from build123d import *

# Parameters (mm, degrees)
SKETCH1_R           = 3
BOSS_EXTRUDE1_DEPTH = 1.5
SKETCH2_R           = 1.875
BOSS_EXTRUDE2_DEPTH = 15
CUT_EXTRUDE1_DEPTH  = 0.75
FILLET2_R           = 0.1


with BuildPart() as part:
    # Sketch1 → Boss-Extrude1 (new body)
    with BuildSketch(Plane.XY):
        Circle(SKETCH1_R)
    extrude(amount=BOSS_EXTRUDE1_DEPTH)

    # Sketch2 → Boss-Extrude2 (add)
    with BuildSketch(Plane.XY.offset(1.5)):
        Circle(SKETCH2_R)
    extrude(amount=BOSS_EXTRUDE2_DEPTH)

    # Sketch3 → Cut-Extrude1 (cut)
    with BuildSketch(Plane(origin=(0, 0, 0), x_dir=(-1, 0, 0), z_dir=(0, 0, -1))):
        with BuildLine():
            Line((2.977836652, 0.322793516), (-2.982583502, 0.322793516))
            ThreePointArc((-2.982583502, 0.322793516), (-3, 0), (-2.982583502, -0.322793516))
            ThreePointArc((-2.982583502, -0.322793516), (-2.980281261, -0.343400064), (-2.977836652, -0.363990208))
            Line((-2.977836652, -0.363990208), (2.977836652, -0.363990208))
            ThreePointArc((2.977836652, -0.363990208), (2.994454037, -0.182332173), (3, 0))
            ThreePointArc((3, 0), (2.995642711, 0.161631516), (2.982583502, 0.322793516))
            Line((2.982583502, 0.322793516), (2.977836652, 0.322793516))
        make_face()
    extrude(amount=-CUT_EXTRUDE1_DEPTH, mode=Mode.SUBTRACT)

    # Fillet2
    fillet2_edges = [part.edges().sort_by_distance(p)[0] for p in [
        (0, -0.363990208, 0.75),
        (0, 0.322793516, 0.75),
    ]]
    fillet(fillet2_edges, radius=FILLET2_R)


solid = part.part
Check sheet for the modelled part. Datum: model origin and axes. Units: mm. A direction names the side the tool comes from. Round coordinates to 2 decimals unless told otherwise and drop trailing zeros. Order: outer loops, then holes, each group sorted by start corner. A loop starts at its lowest first (then second) coordinate and runs counter-clockwise, first axis right, second up.
(1) Access from +Z, -Z, +X, -X, +Y, -Y to the whole of each face (thin tool, end or side, straight path). Record for faces 1 (the cylindrical face through (-1.873, 0.082, 8.895)), 2 (the flat face through (0, -1, 0)).
(2) Cross-section at A-A, the plane y = 0. Enter the section's corners in (x, z) (3 decimals), and give its area (4 significant figures).
(3) Scan lines: probe 1 along Z at (x, y) = (-1.5, 1.5); probe 2 along Z at (x, y) = (-1, 0.25); probe 3 along Y at (x, z) = (0.5, 14.75). Record each from-to range of solid material in increasing order.
(4) Cross-section at C-C, the plane z = 11.5. Enter the section's corners in (x, y) (3 decimals), and give its area (3 significant figures).
(5) Cross-section at D-D, the plane y = 1. Enter the section's corners in (x, z), and give its area (3 significant figures).
(6) Cross-section at B-B, the plane x = 0. Enter the section's corners in (y, z) (3 decimals).
(7) Go/stop test with flat-tipped pins: P1, Ø1, axis at x = -0.5, z = 6.5, coming from the +Y side (3 decimals); P2, Ø3, axis at y = 0.5, z = 11, coming from the +X side (3 decimals); P3, Ø1, axis at y = 1, z = 13, coming from the -X side. Record where each tip stops, or that it passes through.
Check sheet entries:
1. face 1: +Z
1. face 2: -Z, +X, -X, +Y, -Y
2. outline: (-3, 0.75) - (3, 0.75) - (3, 1.5) - (1.875, 1.5) - (1.875, 16.5) - (-1.875, 16.5) - (-1.875, 1.5) - (-3, 1.5) - close
2. area: 60.75 mm2
3. probe 1: z = 0 to 1.5
3. probe 2: z = 0.75 to 16.5
3. probe 3: y = -1.81 to 1.81
4. outline: circle Ø3.75 at (0, 0)
4. area: 11.0 mm2
5. outline: (-2.83, 0) - (2.83, 0) - (2.83, 1.5) - (1.59, 1.5) - (1.59, 16.5) - (-1.59, 16.5) - (-1.59, 1.5) - (-2.83, 1.5) - close
5. area: 56.1 mm2
6. outline: (-3, 0) - (-0.364, 0) - (-0.364, 0.65) arc R0.1 cw to (-0.264, 0.75) - (0.223, 0.75) arc R0.1 cw to (0.323, 0.65) - (0.323, 0) - (3, 0) - (3, 1.5) - (1.875, 1.5) - (1.875, 16.5) - (-1.875, 16.5) - (-1.875, 1.5) - (-3, 1.5) - close
7. P1: stops at y = 1.875
7. P2: stops at x = 1.875
7. P3: stops at x = -1.81
